Check sheet for the modelled part. Datum: model origin and axes. Units: mm. Round coordinates to 2 decimals unless told otherwise and drop trailing zeros. Order: outer loops, then holes, each group sorted by start corner. A loop starts at its lowest first (then second) coordinate and runs counter-clockwise, first axis right, second up. Notation, with made-up numbers: (49.5, -9.75) -> (90.5, -9.75) arc R27 cw to (90.5, 26.25) -> close; hole circle Ø1 at (60.25, 24.25). An arc over 180 degrees is marked (long way). Answer in a Markdown table with one row per item.
```python
from build123d import *

# Parameters (mm, degrees)
SCHIZZO1_W                   = 150
SCHIZZO1_H                   = 150
ESTRUSIONE_ESTRUSIONE1_DEPTH = 0.5
RACCORDO1_R                  = 10
FORO_PER_VITE_M5_1_D         = 5.5
SCHIZZO3_W                   = 37.184364996
SCHIZZO3_H                   = 23.849136367
TAGLIO_ESTRUSIONE1_DEPTH     = 1


with BuildPart() as part:
    # Schizzo1 → Estrusione-Estrusione1 (new body)
    with BuildSketch(Plane.XY):
        Rectangle(SCHIZZO1_W, SCHIZZO1_H)
    extrude(amount=ESTRUSIONE_ESTRUSIONE1_DEPTH)

    # Raccordo1
    raccordo1_edges = [part.edges().sort_by_distance(p)[0] for p in [
        (75, -75, 0.25),
        (-75, -75, 0.25),
        (-75, 75, 0.25),
        (75, 75, 0.25),
    ]]
    fillet(raccordo1_edges, radius=RACCORDO1_R)

    # Foro per Vite M5-1 (through all)
    with Locations(Plane(origin=(-48.17969376, -41.96615453, 0.5), x_dir=(1, 0, 0), z_dir=(0, 0, 1))):
        with Locations((0, 0), (23.145595818, 39.745135108), (78.516154922, 58.824197627), (87.390661123, 7.359607969), (11.313576068, 86.409501177), (86.764478148, 97.604587147), (49.762627912, 77.691347737)):
            Hole(FORO_PER_VITE_M5_1_D / 2)

    # Schizzo3 → Taglio-Estrusione1 (cut)
    with BuildSketch(Plane.XY.offset(0.5)):
        with Locations((0, -35.505311098)):
            Rectangle(SCHIZZO3_W, SCHIZZO3_H)
    extrude(amount=-TAGLIO_ESTRUSIONE1_DEPTH, mode=Mode.SUBTRACT)


solid = part.part
```
(1) Draft check along Y on faces 1 (the cylindrical face through (-50.803, -41.14, 0.246)), 2 (the flat face through (-1, 1, 0.5)), 3 (the cylindrical face through (-34.84, 46.3, 0.25)), 4 (the cylindrical face through (-72.15, 71.99, 0.25)). Enter one of: pulls with the +Y half, pulls with the -Y half, needs draft (parallel to the pull), parting line crosses it, or undercut.
Solutions:
| item | result |
|---|---|
| face 1 | undercut |
| face 2 | needs draft |
| face 3 | undercut |
| face 4 | pulls with the +Y half |
(2) Section check A-A on x = -4.5. Record the boundary of the cut face in (y, z).
Solutions:
| item | result |
|---|---|
| outline | (-75, 0) -> (-47.43, 0) -> (-47.43, 0.5) -> (-75, 0.5) -> close; (-23.58, 0) -> (75, 0) -> (75, 0.5) -> (-23.58, 0.5) -> close |
(3) Section check C-C on x = -36.5. Record the boundary of the cut face in (y, z).
Solutions:
| item | result |
|---|---|
| outline | (-75, 0) -> (41.72, 0) -> (41.72, 0.5) -> (-75, 0.5) -> close; (47.17, 0) -> (75, 0) -> (75, 0.5) -> (47.17, 0.5) -> close |
(4) Scan lines: probe 1 along X at (y, z) = (-46, 0.4); probe 2 along Y at (x, z) = (7.5, 0.4); probe 3 along X at (y, z) = (-37, 0.3). Record each from-to range of solid material in increasing order. Write a range as from..to.
Solutions:
| item | result |
|---|---|
| probe 1 | -75..-18.59, 18.59..75 |
| probe 2 | -75..-47.43, -23.58..75 |
| probe 3 | -75..-18.59, 18.59..37.86, 40.57..75 |
(5) Depth check by flat-ended pin: pin 1 Ø5 at (x, y) = (2.5, 30.5) entering from -Z; pin 2 Ø4.5 at (x, y) = (38.58, 55.64) entering from -Z. Enter the tip coordinate at first touch or a pass-through.
Solutions:
| item | result |
|---|---|
| pin 1 | z = 0 |
| pin 2 | through |
(6) Section check B-B on z = 0.4. Give the number of separate pieces and of enclosed holes in the cut face, plus the area to 3 significant figures.
Solutions:
| item | result |
|---|---|
| separate pieces | 1 |
| enclosed holes | 8 |
| area | 21,400 mm^2 |
